```python
from build123d import *

# Parameters (mm, degrees)
BOSS_EXTRUDE1_DEPTH = 25
CUT_EXTRUDE1_DEPTH  = 56
CUT_EXTRUDE2_DEPTH  = 2
CUT_EXTRUDE3_DEPTH  = 56.0000001
BOSS_EXTRUDE2_DEPTH = 0.5
FILLET2_R           = 5
FILLET4_R           = 5
FILLET5_R           = 5
SKETCH6_R           = 4
SKETCH6_R_2         = 2.5
SKETCH6_R_3         = 1.5
SKETCH6_W           = 7
SKETCH6_H           = 1.501556971
CUT_EXTRUDE4_DEPTH  = 1
BOSS_EXTRUDE3_DEPTH = 0.5
SKETCH8_R           = 0.5
BOSS_EXTRUDE4_DEPTH = 0.5
CUT_EXTRUDE5_DEPTH  = 0.5
SKETCH10_W          = 2
SKETCH10_H          = 4
BOSS_EXTRUDE5_DEPTH = 0.5
CUT_EXTRUDE6_DEPTH  = 2
CUT_EXTRUDE7_DEPTH  = 2


with BuildPart() as part:
    # Sketch1 → Boss-Extrude1 (new body)
    with BuildSketch(Plane(origin=(0, 0, 0), x_dir=(1, 0, 0), z_dir=(0, 1, 0))):
        with BuildLine():
            Line((-27.5, 6.25), (-27.5, -15))
            Line((-27.5, -15), (27.5, -15))
            Line((27.5, -15), (27.5, 6.25))
            ThreePointArc((27.5, 6.25), (0, 15), (-27.5, 6.25))
        make_face()
    extrude(amount=BOSS_EXTRUDE1_DEPTH)

    # Sketch2 → Cut-Extrude1 (cut, through all)
    with BuildSketch(Plane(origin=(27.5, 0, 0), x_dir=(0, 0, -1), z_dir=(1, 0, 0))):
        Polygon((-15, 8), (15, 22.824529963), (15, 25), (-15, 25), align=None)
    extrude(amount=-CUT_EXTRUDE1_DEPTH, mode=Mode.SUBTRACT)

    # Sketch3 → Cut-Extrude2 (cut)
    with BuildSketch(Plane(origin=(0, 12.387436262, 6.121264001), x_dir=(1, 0, 0), z_dir=(0, 0.89651484, 0.443013704))):
        with BuildLine():
            Line((-25.5, 10.23830007), (-25.5, -7.903612972))
            Line((-25.5, -7.903612972), (25.5, -7.903612972))
            Line((25.5, -7.903612972), (25.5, 10.238296947))
            ThreePointArc((25.5, 10.238296947), (24.907293379, 12.599602744), (23.269693973, 14.40108391))
            add(Edge.make_bspline(
                [(23.269693973, 14.40108391), (22.122214348, 15.164554976), (20.94493023, 15.871336285), (17.734831315, 17.599553604), (15.649676942, 18.521436915), (12.93284925, 19.463833346), (12.383197637, 19.641920344), (11.282858983, 19.973451503), (10.731016127, 20.127331411), (9.070515859, 20.553661297), (7.956893593, 20.790850084), (4.596297841, 21.362298201), (2.329710672, 21.557257961), (-1.110917839, 21.560300401), (-2.268023373, 21.512162029), (-4.552325625, 21.320060503), (-5.684502339, 21.176395804), (-9.051900597, 20.606337494), (-11.258147255, 20.041629121), (-14.509660741, 18.918382275), (-15.58692593, 18.496052007), (-17.688755449, 17.572497213), (-18.716963562, 17.07031031), (-20.937080939, 15.876150048), (-22.119122989, 15.166616669), (-23.269698352, 14.40108412)],
                knots=[0.04966081, 0.04966081, 0.04966081, 0.04966081, 0.125, 0.125, 0.25, 0.25, 0.28125, 0.28125, 0.3125, 0.3125, 0.375, 0.375, 0.5, 0.5, 0.5625, 0.5625, 0.625, 0.625, 0.75, 0.75, 0.8125, 0.8125, 0.875, 0.875, 0.950394251, 0.950394251, 0.950394251, 0.950394251], degree=3))
            ThreePointArc((-23.269698352, 14.40108412), (-24.907294621, 12.599603549), (-25.5, 10.23830007))
        make_face()
    extrude(amount=-CUT_EXTRUDE2_DEPTH, mode=Mode.SUBTRACT)

    # Sketch4 → Cut-Extrude3 (cut, through all)
    with BuildSketch(Plane(origin=(27.5, 0, 0), x_dir=(0, 0, -1), z_dir=(1, 0, 0))):
        Polygon((-15, 8), (-15, 6), (6.25, 18.500708724), align=None)
    extrude(amount=-CUT_EXTRUDE3_DEPTH, mode=Mode.SUBTRACT)

    # Sketch5 → Boss-Extrude2 (add)
    with BuildSketch(Plane(origin=(0, 10.594406582, 5.235236594), x_dir=(1, 0, 0), z_dir=(0, 0.89651484, 0.443013704))):
        with BuildLine():
            Line((-21.874738248, 1.358474377), (-21.874738248, -0.903612972))
            ThreePointArc((-21.874738248, -0.903612972), (-20.410272153, -4.439146877), (-16.874738248, -5.903612972))
            Line((-16.874738248, -5.903612972), (17.125261752, -5.903612972))
            ThreePointArc((17.125261752, -5.903612972), (20.660795658, -4.439146877), (22.125261752, -0.903612972))
            Line((22.125261752, -0.903612972), (22.125261752, 1.358474377))
            Line((22.125261752, 1.358474377), (19.047514764, 12.900025582))
            ThreePointArc((19.047514764, 12.900025582), (16.54852317, 16.647309018), (12.283870187, 18.096387028))
            Line((12.283870187, 18.096387028), (-12.033346682, 18.096387028))
            ThreePointArc((-12.033346682, 18.096387028), (-16.297999665, 16.647309018), (-18.796991259, 12.900025582))
            Line((-18.796991259, 12.900025582), (-21.874738248, 1.358474377))
        make_face()
        with BuildLine():
            Line((-16.874738248, -3.903612972), (17.125261752, -3.903612972))
            ThreePointArc((17.125261752, -3.903612972), (19.246582096, -3.024933315), (20.125261752, -0.903612972))
            Line((20.125261752, -0.903612972), (20.125261752, 1.096387028))
            Line((20.125261752, 1.096387028), (17.115044885, 12.384700281))
            ThreePointArc((17.115044885, 12.384700281), (15.330050889, 15.061331307), (12.283870187, 16.096387028))
            Line((12.283870187, 16.096387028), (-12.033346682, 16.096387028))
            ThreePointArc((-12.033346682, 16.096387028), (-15.079527384, 15.061331307), (-16.86452138, 12.384700281))
            Line((-16.86452138, 12.384700281), (-19.874738248, 1.096387028))
            Line((-19.874738248, 1.096387028), (-19.874738248, -0.903612972))
            ThreePointArc((-19.874738248, -0.903612972), (-18.996058591, -3.024933315), (-16.874738248, -3.903612972))
        make_face(mode=Mode.SUBTRACT)
    extrude(amount=BOSS_EXTRUDE2_DEPTH)

    # Fillet2
    fillet2_edges = [part.edges().sort_by_distance(p)[0] for p in [
        (-27.5, 9.250354362, -6.25),
        (27.5, 9.250354362, -6.25),
    ]]
    fillet(fillet2_edges, radius=FILLET2_R)

    # Fillet4
    fillet4_edges = [part.edges().sort_by_distance(p)[0] for p in [
        (27.5, 3, 15),
        (-27.5, 3, 15),
    ]]
    fillet(fillet4_edges, radius=FILLET4_R)

    # Fillet5
    fillet5_edges = [part.edges().sort_by_distance(p)[0] for p in [
        (25.5, 7.280109363, 12.413404314),
        (-25.5, 7.280109363, 12.413404314),
    ]]
    fillet(fillet5_edges, radius=FILLET5_R)

    # Sketch6 → Cut-Extrude4 (cut)
    with BuildSketch(Plane(origin=(0, 10.594406582, 5.235236594), x_dir=(1, 0, 0), z_dir=(0, 0.89651484, 0.443013704))):
        with Locations((-7.391955117, 9.096387028)):
            Circle(SKETCH6_R)
        with Locations((7.642478622, 9.096387028)):
            Circle(SKETCH6_R)
        with Locations((-14.246179645, 6.679307091)):
            Circle(SKETCH6_R_2)
        with Locations((-16.626340028, 0.096387028)):
            Circle(SKETCH6_R_2)
        with Locations((-9.933747273, 0.096387028)):
            Circle(SKETCH6_R_2)
        with Locations((10.184270778, 0.096387028)):
            Circle(SKETCH6_R_2)
        with Locations((16.876863533, 0.096387028)):
            Circle(SKETCH6_R_2)
        with Locations((14.49670315, 6.679307091)):
            Circle(SKETCH6_R_2)
        with Locations((0.125261752, 6.096387028)):
            Circle(SKETCH6_R_3)
        with Locations((0.125261752, 2.372758697)):
            Rectangle(SKETCH6_W, SKETCH6_H)
    extrude(amount=-CUT_EXTRUDE4_DEPTH, mode=Mode.SUBTRACT)

    # Sketch7 → Boss-Extrude3 (add)
    with BuildSketch(Plane(origin=(0, 9.697891742, 4.79222289), x_dir=(1, 0, 0), z_dir=(0, 0.89651484, 0.443013704))):
        with BuildLine():
            Line((-8.048414678, 9.459100199), (-9.681837773, 6.502835312))
            Line((-9.681837773, 6.502835312), (-6.950708776, 8.489920486))
            ThreePointArc((-6.950708776, 8.489920486), (-6.895561612, 9.65860895), (-8.048414678, 9.459100199))
        make_face()
        with BuildLine():
            Line((8.298938183, 9.459100199), (9.932361278, 6.502835312))
            Line((9.932361278, 6.502835312), (7.201232281, 8.489920486))
            ThreePointArc((7.201232281, 8.489920486), (7.146085117, 9.65860895), (8.298938183, 9.459100199))
        make_face()
    extrude(amount=BOSS_EXTRUDE3_DEPTH)

    # Sketch8 → Boss-Extrude4 (add)
    with BuildSketch(Plane(origin=(0, 9.697891742, 4.79222289), x_dir=(1, 0, 0), z_dir=(0, 0.89651484, 0.443013704))):
        with Locations((-14.246179645, 6.679307091)):
            Circle(SKETCH8_R)
        with Locations((-16.626340028, 0.096387028)):
            Circle(SKETCH8_R)
        with Locations((-9.933747273, 0.096387028)):
            Circle(SKETCH8_R)
        with Locations((14.49670315, 6.679307091)):
            Circle(SKETCH8_R)
        with Locations((10.184270778, 0.096387028)):
            Circle(SKETCH8_R)
        with Locations((16.876863533, 0.096387028)):
            Circle(SKETCH8_R)
    extrude(amount=BOSS_EXTRUDE4_DEPTH)

    # Sketch9 → Cut-Extrude5 (cut)
    with BuildSketch(Plane(origin=(0, 9.697891742, 4.79222289), x_dir=(1, 0, 0), z_dir=(0, 0.89651484, 0.443013704))):
        Polygon((-9.58567888, 6.572797555), (-8.049200513, 7.690691798), (-5.371486784, 7.690691798), (-5.371486784, 6.572797555), align=None)
    extrude(amount=-CUT_EXTRUDE5_DEPTH, mode=Mode.SUBTRACT)

    # Sketch10 → Boss-Extrude5 (add)
    with BuildSketch(Plane(origin=(0, 10.594406582, 5.235236594), x_dir=(1, 0, 0), z_dir=(0, 0.89651484, 0.443013704))):
        with Locations((-22.660381166, 8.906356756)):
            Rectangle(SKETCH10_W, SKETCH10_H)
        with Locations((23.5, 8.906356756)):
            Rectangle(SKETCH10_W, SKETCH10_H)
    extrude(amount=BOSS_EXTRUDE5_DEPTH)

    # Sketch11 → Cut-Extrude6 (cut)
    with BuildSketch(Plane.ZY.offset(-22.5)):
        Polygon((-4.320967236, 15.874329501), (-0.923579886, 13.720464249), (-0.734907876, 14.102274687), align=None)
    extrude(amount=-CUT_EXTRUDE6_DEPTH, mode=Mode.SUBTRACT)

    # Sketch12 → Cut-Extrude7 (cut)
    with BuildSketch(Plane.ZY.offset(23.660381166)):
        Polygon((-4.320967236, 15.874329501), (-0.956414728, 13.654017267), (-0.734907876, 14.102274687), align=None)
    extrude(amount=-CUT_EXTRUDE7_DEPTH, mode=Mode.SUBTRACT)


solid = part.part
```
Build history of the part. All positions in model axes, mm. A direction names the side the tool comes from. Give positions to 0.01 mm unless a question says otherwise; leave off trailing zeros. Write item = value, one per line. Start each with the question number.
(1) Probe L1, parallel to X at y = 12.75, z = 0; L2, parallel to Y at x = 11, z = -8; L3, parallel to X at y = 16.75, z = -6. List the from-to ranges inside material, lowest first. Write a range as [from, to].
(2) Two-plate mould, pull along Z, no slides. Class faces 1 (the cylindrical face through (-6.882, 14.192, -3.746)), 2 (the cylindrical face through (26.853, 9.772, -6.031)), 3 (the cylindrical face through (-20.45, 8.87, 9.29)): released by +Z, released by -Z, zero draft, split by the parting line, or undercut.
(3) Which spindle directions (+Z, -Z, +X, -X, +Y, -Y) get a long thin tool onto all of the face, cutting with end or side? Do faces 4 (the cylindrical face through (-19.019, 9.486, 8.035)), 5 (the flat face through (-13.726, 12.426, -0.729)), 6 (the flat face through (-21.875, 11, 5)), 7 (the flat face through (-18.35, 13.84, -0.77)). Say none if no direction does.
(4) Pin check, flat tips, straight feed: pin 1 Ø1.5 at (x, y) = (-16.5, 14) entering from +Z; pin 2 Ø2 at (y, z) = (14, -6) entering from +X; pin 3 Ø12 at (x, z) = (-16, -11) entering from +Y. Stop position of each tip, or through.
Responses:
q1.L1 = [-27.5, -16.52], [-11.97, -9.42], [-5.36, -1.31], [1.56, 5.61], [9.67, 12.22], [16.77, 27.5]
q1.L2 = [0, 17.13]
q1.L3 = [-26.87, -24.79], [24.79, 26.87]
q2.face_1 = undercut
q2.face_2 = released by -Z
q2.face_3 = released by +Z
q3.face_4 = +Y
q3.face_5 = none
q3.face_6 = +Z, +Y
q3.face_7 = +Z
q4.pin_1 = -0.17
q4.pin_2 = 27.29
q4.pin_3 = 22.22
